Geometry: see drawing. Coordinates: mm, zero at the bounding-box minimum. A direction names the side the tool comes from. Give positions to 0.01 mm unless a question says otherwise; leave off trailing zeros. Write each loop counter-clockwise with the first axis right and the second up, starting at its lowest first coordinate (ties: lowest second). Pieces come first, ordered by that corner, then holes. Notation, with made-up numbers: M 71.25,49 L 90.25,49 A19 cw 90.25,72 Z; hole C 65.25,43.25 d11. An arc over 180 degrees is marked long. Use a Markdown table: item, result. Add a question column.
1) Section C-C on x = 20. Return the cut outline in (y, z).
2) Set-up query: the marked faces 1 and 2. Return all of +Z, -Z, +X, -X, +Y, -Y with unobstructed straight access to the full face (end or side cutting, diameter ignored); none if empty.
3) Pin query (flat end, axial travel): pin 1 (1.5 mm diameter, centred on x = 14.5, z = 11, fed in from +Y); pin 2 (8 mm diameter, centred on y = 8, z = 50.5, fed in from +X). Return the tip coordinate at first contact, or that it passes through.
4) Section B-B on y = 12.5. Return the cut outline in (x, z), then the cut area to 3 significant figures.
5) Line query: line 1 (Z direction, x = 34, y = 4); line 2 (Y direction, x = 26, z = 17.5). Output: solid intervals per line, ascending.
6) Section D-D on y = 23.25. Return the cut outline in (x, z), then the cut area to 3 significant figures.
7) Section A-A on z = 35. Return the cut outline in (x, y), then the cut area to 3 significant figures.
8) Draft query along Z for the marked faces 3, 4, 5 and 6. Return one class per face: +Z half, -Z half, draft (parallel to the pull), parting line (faces both ways), or undercut.
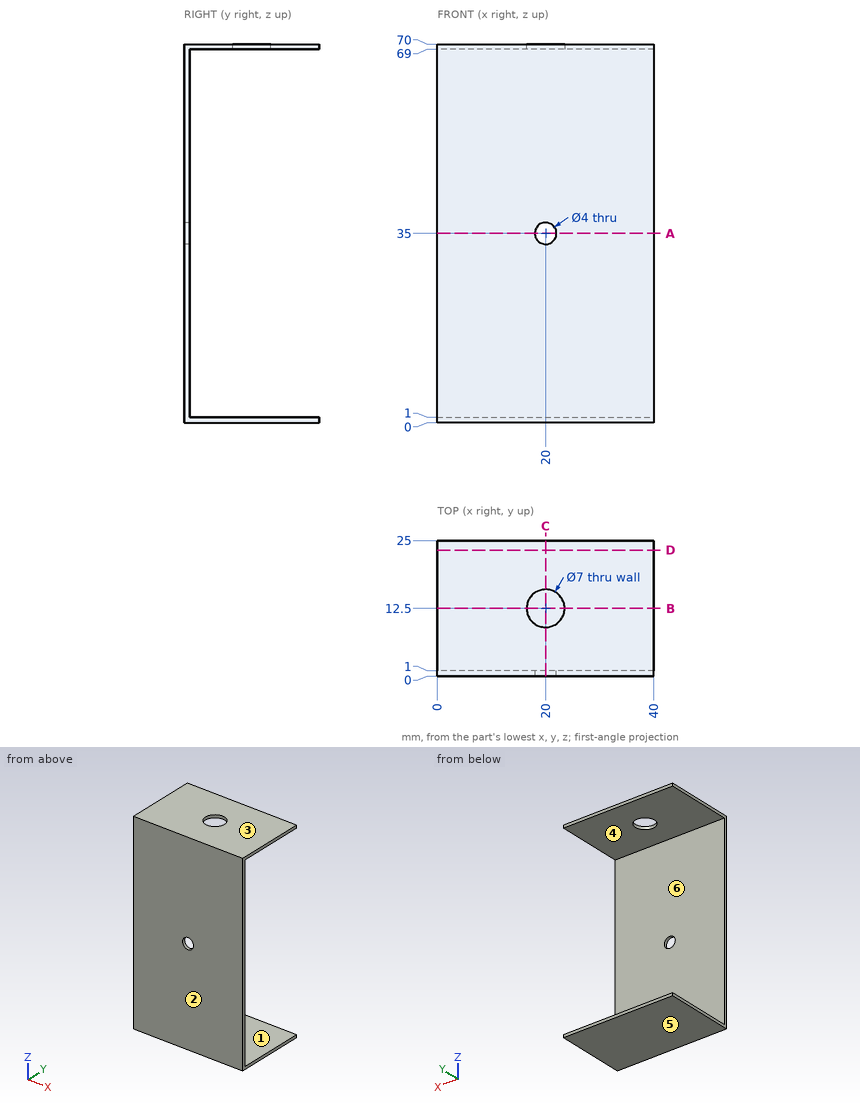
Found:
| question | item | result |
|---|---|---|
| 1 | outline | M 0,0 L 25,0 L 25,1 L 1,1 L 1,33 L 0,33 Z; M 0,37 L 1,37 L 1,69 L 9,69 L 9,70 L 0,70 Z; M 16,69 L 25,69 L 25,70 L 16,70 Z |
| 2 | face 1 | +X, -X, +Y |
| 2 | face 2 | +Z, -Z, +X, -X, -Y |
| 3 | pin 1 | y = 1 |
| 3 | pin 2 | through |
| 4 | outline | M 0,0 L 40,0 L 40,1 L 0,1 Z; M 0,69 L 16.5,69 L 16.5,70 L 0,70 Z; M 23.5,69 L 40,69 L 40,70 L 23.5,70 Z |
| 4 | area | 73.0 mm² |
| 5 | line 1 | 0 to 1, 69 to 70 |
| 5 | line 2 | 0 to 1 |
| 6 | outline | M 0,0 L 40,0 L 40,1 L 0,1 Z; M 0,69 L 40,69 L 40,70 L 0,70 Z |
| 6 | area | 80.0 mm² |
| 7 | outline | M 0,0 L 18,0 L 18,1 L 0,1 Z; M 22,0 L 40,0 L 40,1 L 22,1 Z |
| 7 | area | 36.0 mm² |
| 8 | face 3 | +Z half |
| 8 | face 4 | undercut |
| 8 | face 5 | -Z half |
| 8 | face 6 | undercut |
